Input: part model. Units: mm. Frame: model coordinates. Give positions to 0.01 mm unless a question says otherwise; leave off trailing zeros. Order: outer loops, then holes, each group sorted by start corner. A loop starts at its lowest first (then second) coordinate and runs counter-clockwise, first axis right, second up.
Autodesk Inventor part; units mm, degrees
ref_plane "YZ Plane" through (0, 0, 0) normal (1, 0, 0) x (0, 1, 0)
ref_plane "XZ Plane" through (0, 0, 0) normal (0, 1, 0) x (-1, 0, 0)
ref_plane "XY Plane" through (0, 0, 0) normal (0, 0, 1) x (1, 0, 0)
sketch "Sketch2" plane through (0, 0, 0) normal (1, 0, 0) x (0, 1, 0)
  line L0 (-2.5, 55.99) -> (-2.5, 18.99)
  line L1 (-2.5, 18.99) -> (-150.5, 18.99)
  line L2 (-150.5, 18.99) -> (-150.5, 55.99)
  line L3 (-150.5, 55.99) -> (-2.5, 55.99)
  line L4 (87, 57.49) -> (-160.5, 57.49)
  line L5 (-151, 57.49) -> (-2, 57.49)
  line L6 (-2, 57.49) -> (-2, 17.99)
  line L7 (-2, 17.99) -> (-151, 17.99)
  line L8 (-151, 17.99) -> (-151, 57.49)
  dimension "d1" = 1.5
  dimension "d2" = 0.5
  dimension "d3" = 0.5
  dimension "d4" = 1
extrude "Extrusion1" add sketch "Sketch2" along normal blind 2 contours L0 L1 L2 L3 | L6 L7 L8 L4
sketch "Sketch3" plane through (0, 0, 0) normal (-1, 0, 0) x (0, -1, 0)
  arc A0 (111.6743, 41.99) -> (112.6358, 43.2647) centre (111.6743, 42.99) ccw
  line L0 (111.2072, 48.2647) -> (112.6358, 43.2647)
  arc A1 (111.2072, 48.2647) -> (110.2457, 48.99) centre (110.2457, 47.99) ccw
  line L1 (98.7543, 48.99) -> (110.2457, 48.99)
  arc A2 (98.7543, 48.99) -> (97.7928, 48.2647) centre (98.7543, 47.99) ccw
  line L2 (96.3642, 43.2647) -> (97.7928, 48.2647)
  arc A3 (96.3642, 43.2647) -> (97.3257, 41.99) centre (97.3257, 42.99) ccw
  line L3 (111.6743, 41.99) -> (97.3257, 41.99)
  circle A4 centre (114.8571, 45.99) radius 0.7915
  circle A5 centre (94.1429, 45.99) radius 0.7915
  line L4 (143.6743, 41.99) -> (129.3257, 41.99)
  arc A6 (128.3642, 43.2647) -> (129.3257, 41.99) centre (129.3257, 42.99) ccw
  line L5 (128.3642, 43.2647) -> (129.7928, 48.2647)
  arc A7 (130.7543, 48.99) -> (129.7928, 48.2647) centre (130.7543, 47.99) ccw
  line L6 (130.7543, 48.99) -> (142.2457, 48.99)
  arc A8 (143.2072, 48.2647) -> (142.2457, 48.99) centre (142.2457, 47.99) ccw
  line L7 (143.2072, 48.2647) -> (144.6358, 43.2647)
  arc A9 (143.6743, 41.99) -> (144.6358, 43.2647) centre (143.6743, 42.99) ccw
  circle A10 centre (146.8571, 45.99) radius 0.7915
  circle A11 centre (126.1429, 45.99) radius 0.7915
  line L8 (108.7808, 33.99) -> (135.2192, 33.99)
  arc A12 (108.7808, 33.99) -> (107.8106, 33.2325) centre (108.7808, 32.99) ccw
  line L9 (106.3106, 27.2325) -> (107.8106, 33.2325)
  arc A13 (106.3106, 27.2325) -> (107.2808, 25.99) centre (107.2808, 26.99) ccw
  line L10 (136.7192, 25.99) -> (107.2808, 25.99)
  arc A14 (136.7192, 25.99) -> (137.6894, 27.2325) centre (136.7192, 26.99) ccw
  line L11 (136.1894, 33.2325) -> (137.6894, 27.2325)
  arc A15 (136.1894, 33.2325) -> (135.2192, 33.99) centre (135.2192, 32.99) ccw
  circle A16 centre (140, 29.99) radius 0.7915
  circle A17 centre (104, 29.99) radius 0.7915
  arc A18 (95.4027, 43.5394) -> (97.3257, 40.99) centre (97.3257, 42.99) ccw
  line L12 (95.4027, 43.5394) -> (96.8313, 48.5394)
  arc A19 (98.7543, 49.99) -> (96.8313, 48.5394) centre (98.7543, 47.99) ccw
  line L13 (98.7543, 49.99) -> (110.2457, 49.99)
  arc A20 (112.1687, 48.5394) -> (110.2457, 49.99) centre (110.2457, 47.99) ccw
  line L14 (112.1687, 48.5394) -> (113.5973, 43.5394)
  arc A21 (111.6743, 40.99) -> (113.5973, 43.5394) centre (111.6743, 42.99) ccw
  line L15 (111.6743, 40.99) -> (97.3257, 40.99)
  circle A22 centre (94.1429, 45.99) radius 2
  line L16 (94.1429, 47.99) -> (96.6743, 47.99)
  line L17 (94.1429, 43.99) -> (95.5314, 43.99)
  circle A23 centre (114.8571, 45.99) radius 2
  line L18 (114.8571, 47.99) -> (112.3257, 47.99)
  line L19 (114.8571, 43.99) -> (113.4686, 43.99)
  circle A24 centre (126.1429, 45.99) radius 2
  circle A25 centre (146.8571, 45.99) radius 2
  circle A26 centre (140, 29.99) radius 2
  circle A27 centre (104, 29.99) radius 2
  line L20 (142.2457, 49.99) -> (130.7543, 49.99)
  arc A28 (130.7543, 49.99) -> (128.8313, 48.5394) centre (130.7543, 47.99) ccw
  line L21 (128.8313, 48.5394) -> (127.4027, 43.5394)
  arc A29 (127.4027, 43.5394) -> (129.3257, 40.99) centre (129.3257, 42.99) ccw
  line L22 (129.3257, 40.99) -> (143.6743, 40.99)
  arc A30 (143.6743, 40.99) -> (145.5973, 43.5394) centre (143.6743, 42.99) ccw
  line L23 (145.5973, 43.5394) -> (144.1687, 48.5394)
  arc A31 (144.1687, 48.5394) -> (142.2457, 49.99) centre (142.2457, 47.99) ccw
  line L24 (126.1429, 47.99) -> (128.6743, 47.99)
  line L25 (126.1429, 43.99) -> (127.5314, 43.99)
  line L26 (146.8571, 47.99) -> (144.3257, 47.99)
  line L27 (146.8571, 43.99) -> (145.4686, 43.99)
  line L28 (135.2192, 34.99) -> (108.7808, 34.99)
  arc A32 (108.7808, 34.99) -> (106.8405, 33.4751) centre (108.7808, 32.99) ccw
  line L29 (106.8405, 33.4751) -> (105.3405, 27.4751)
  arc A33 (105.3405, 27.4751) -> (107.2808, 24.99) centre (107.2808, 26.99) ccw
  line L30 (107.2808, 24.99) -> (136.7192, 24.99)
  arc A34 (136.7192, 24.99) -> (138.6595, 27.4751) centre (136.7192, 26.99) ccw
  line L31 (138.6595, 27.4751) -> (137.1595, 33.4751)
  arc A35 (137.1595, 33.4751) -> (135.2192, 34.99) centre (135.2192, 32.99) ccw
  line L32 (104, 31.99) -> (106.4692, 31.99)
  line L33 (104, 27.99) -> (105.4692, 27.99)
  line L34 (140, 31.99) -> (137.5308, 31.99)
  line L35 (140, 27.99) -> (138.5308, 27.99)
  dimension "d7" = 1
  dimension "d8" = 4
  dimension "d9" = 1
  dimension "d10" = 1
extrude "Extrusion2" cut sketch "Sketch3" against normal through all contours L3 A3 L2 A2 L1 A1 L0 A0 | A4 | A5 | L4 A6 L5 A7 L6 A8 L7 A9 | A10 | A11 | L8 A15 L11 A14 L10 A13 L9 A12 | A16 | A17 | L12 A22 A19 L13 A20 L14 A23 A21 L15 A18 | L17 A22 L12 | A22 L12 | L12 A22 | A22 L16 L12 | L14 A23 L19 | A23 L14 | L14 A23 | L14 L18 A23 | A24 L21 | L24 L21 A24 | A24 L21 L25 | L21 A28 L20 A31 L23 A25 A30 L22 A29 A24 | A24 L21 | L26 A25 L23 | L23 A25 L27 | L23 A25 | A25 L23 | A26 L31 | A26 L31 L34 | L35 L31 A26 | L31 A26 | A26 L31 A34 L30 A33 L29 A27 A32 L28 A35 | L29 A27 L32 | L33 A27 L29 | L29 A27 | A27 L29
sketch "Sketch4" plane through (0, 0, 0) normal (-1, 0, 0) x (0, -1, 0)
  circle A0 centre (55, 48.99) radius 3.5
  circle A1 centre (63, 42.99) radius 3.5
  circle A2 centre (55, 36.99) radius 3.5
  circle A3 centre (63, 30.99) radius 3.5
  circle A4 centre (55, 24.99) radius 3.5
  circle A5 centre (80, 46.99) radius 6
  circle A6 centre (80, 31.99) radius 6
  circle A7 centre (55, 48.99) radius 4.25
  circle A8 centre (63, 42.99) radius 4.25
  circle A9 centre (55, 36.99) radius 4.25
  circle A10 centre (55, 24.99) radius 4.25
  circle A11 centre (63, 30.99) radius 4.25
  circle A12 centre (80, 31.99) radius 7
  circle A13 centre (80, 46.99) radius 7
  dimension "d13" = 8.5
  dimension "d14" = 14
extrude "Extrusion3" cut sketch "Sketch4" against normal through all contours A0 | A1 | A2 | A3 | A4 | A5 | A6 | A7 | A8 | A9 | A10 | A11 | A12 | A13
sketch "Sketch5" plane through (0, 0, 0) normal (-1, 0, 0) x (0, -1, 0)
  line L0 (2, 57.49) -> (151, 57.49)
  line L1 (2, 17.99) -> (2, 57.49)
  line L2 (2, 24.99) -> (22.5, 24.99)
  line L3 (22.5, 24.99) -> (22.5, 57.49)
  line L4 (22.5, 57.49) -> (2, 57.49)
  line L5 (2, 57.49) -> (2, 24.99)
  line L6 (25.5, 21.99) -> (42.5, 21.99)
  line L7 (42.5, 21.99) -> (42.5, 57.49)
  line L8 (42.5, 57.49) -> (25.5, 57.49)
  line L9 (25.5, 57.49) -> (25.5, 21.99)
  line L10 (151, 17.99) -> (2, 17.99)
  dimension "d24" = 4
  dimension "d25" = 7
  dimension "d26" = 20.5
  dimension "d27" = 3
  dimension "d28" = 17
extrude "Extrusion4" cut sketch "Sketch5" against normal through all
equation "\"d9\" = d7"
equation "\"d10\" = d7"
properties part number "config - casing - module protector"
1) Cut plane C-C (y = -12). Return the cut outline in (x, z), then the cut area to 3 significant figures.
2) Cut plane D-D (x = 0.95). Count the separate pieces of the cut face and the enclosed holes in it, then the cut area to 3 significant figures.
3) Pull-direction query (Y, two-part tool) for faces 1 (the face through (0, -94, 38)), 2 (the face through (0.986, -59.054, 50.267)); classes: pulls with the +Y half, pulls with the -Y half, needs draft (parallel to the pull), parting line crosses it, or undercut.
4) Line query: probe 1 along Z at (x, y) = (1.6, -140); probe 2 along Z at (x, y) = (1.5, -63); probe 3 along Z at (x, y) = (0.75, -55). Output: solid intervals per line, ascending.
5) First-contact query: P1, Ø7, axis at y = -55, z = 36.99, coming from the -X side; P2, Ø10, axis at y = -55, z = 48.99, coming from the +X side. Flat tips, straight axial feed; report the tip coordinate or a pass-through.
6) Cut plane B-B (y = -84). Return the cut outline in (x, z).
7) Cut plane A-A (y = -55). Return the cut outline in (x, z).
Geometry says:
1. outline: (0, 17.99) - (2, 17.99) - (2, 24.99) - (0, 24.99) - close
1. area: 14.0 mm2
2. separate pieces: 1
2. enclosed holes: 10
2. area: 3,320 mm2
3. face 1: needs draft
3. face 2: undercut
4. probe 1: z = 17.99 to 27.99, 31.99 to 40.99, 49.99 to 57.49
4. probe 2: z = 17.99 to 26.74, 35.24 to 38.74, 47.24 to 57.49
4. probe 3: z = 17.99 to 20.74, 29.24 to 32.74, 41.24 to 44.74, 53.24 to 57.49
5. P1: passes through
5. P2: stops at x = 2
6. outline: (0, 17.99) - (2, 17.99) - (2, 26.25) - (0, 26.25) - close; (0, 37.73) - (2, 37.73) - (2, 41.25) - (0, 41.25) - close; (0, 52.73) - (2, 52.73) - (2, 57.49) - (0, 57.49) - close
7. outline: (0, 17.99) - (2, 17.99) - (2, 20.74) - (0, 20.74) - close; (0, 29.24) - (2, 29.24) - (2, 32.74) - (0, 32.74) - close; (0, 41.24) - (2, 41.24) - (2, 44.74) - (0, 44.74) - close; (0, 53.24) - (2, 53.24) - (2, 57.49) - (0, 57.49) - close
